Design review of the part built by this model. Coordinates are the model's own, in mm. A direction names the side the tool comes from. Round coordinates to 2 decimals unless told otherwise and drop trailing zeros. Write each loop counter-clockwise with the first axis right and the second up, starting at its lowest first coordinate (ties: lowest second). Pieces come first, ordered by that corner, then holes. Notation, with made-up numbers: M 35.25,30 L 86.25,30 A22 ccw 86.25,64 Z; hole C 32,4.5 d7. An arc over 180 degrees is marked long. One line per question, with ' | ' between items. Start each with the question number.
Item 1: Insertion check: pin 1 Ø2 at (y, z) = (23.5, -4) entering from +X; pin 2 Ø6 at (y, z) = (9.5, 12) entering from +X; pin 3 Ø3 at (y, z) = (3.5, 12.5) entering from -X. Each pin has a flat end and moves straight along its axis. Give the tip position at first contact, or say it passes through.
Item 2: For L1, parallel to Z at x = 7, y = 10; L2, parallel to Z at x = -12.5, y = 11; L3, parallel to X at y = 29, z = -7, list the stretches that pass through material, from the lowest coordinate up.
Item 3: Draft analysis for pull direction Z (two halves, no side actions). For faces 1 (the face through (27.5, 14, -16)), 2 (the face through (28, 19, 21)), 3 (the face through (7.454, 3, 4)), state which applies: released by +Z, released by -Z, zero draft, split by the parting line, or undercut.
Item 4: Add section A-A, the plane x = 0. State the section outline as (y, z) points, and give its area (3 significant figures).
Item 5: Machinability: for faces 4 (the face through (27.5, 14, 16)), 5 (the face through (7.454, 3, -26)), which of the approach directions +Z, -Z, +X, -X, +Y, -Y give a long, thin tool a straight path to every point of the face, cutting with its end or side? Answer none if there is none.
Item 6: Add section B-B, the plane z = 0. State the section outline as (x, y) points, and give its area (3 significant figures).
Item 7: Add section C-C, the plane x = -21. State the section outline as (y, z) points, and give its area (3 significant figures).
Item 8: Add section D-D, the plane y = 41. State the section outline as (x, z) points, and give its area (3 significant figures).
Autodesk Inventor part; units mm, degrees
ref_plane "YZ Plane" through (0, 0, 0) normal (1, 0, 0) x (0, 1, 0)
sketch "Sketch1" plane through (0, 0, 0) normal (0, 1, 0) x (-1, 0, 0)
  circle A0 centre (0, 0) radius 35
  dimension "d0" = 70
extrude "Extrusion1" add sketch "Sketch1" along normal blind 50
sketch "Sketch2" plane through (0, 0, 0) normal (1, 0, 0) x (0, 1, 0)
  point P0 (0, 0)
sketch "Sketch3" plane through (0, 0, 0) normal (0, 0, 1) x (1, 0, 0)
  line L0 (35, 50) -> (-35, 50)
  arc A0 (-35, 50) -> (35, 50) centre (0, 50) ccw
  point P0 (0, 0)
  dimension "d3" = 35
extrude "Extrusion2" cut sketch "Sketch3" against normal blind 50 and the other way blind 50
sketch "Sketch4" plane through (0, 0, 0) normal (0, 0, 1) x (1, 0, 0)
  arc A0 (7.4545, 6.2837) -> (-7.5, 5.4589) centre (0, 5.4589) ccw
  line L0 (7.4545, 6.2837) -> (7.4545, 0)
  line L1 (-35, 0) -> (35, 0)
  line L2 (-7.5, 5.4589) -> (-7.5, 0)
  line L3 (-7.5, 0) -> (7.4545, 0)
  line L4 (7.4545, 0) -> (3.6133, 0)
  line L5 (3.6133, 0) -> (-3.6133, 0)
  line L6 (-3.6133, 0) -> (-7.5, 0)
  point P0 (0, 0)
  dimension "d8" = 15
extrude "Extrusion3" cut sketch "Sketch4" along normal blind 50 and the other way blind 50
sketch "Sketch5" plane through (0, 0, 0) normal (0, 1, 0) x (-1, 0, 0)
  point P0 (0, 0)
sketch "Sketch6" plane through (0, 0, 0) normal (0, 1, 0) x (-1, 0, 0)
  line L0 (-27.5, -2) -> (27.5, -2)
  line L1 (27.5, -2) -> (27.5, 2)
  line L2 (27.5, 2) -> (-27.5, 2)
  line L3 (-27.5, 2) -> (-27.5, -2)
  line L4 (-27.5, -2) -> (27.5, 2) construction
  line L5 (27.5, -2) -> (-27.5, 2) construction
  line L6 (27.5, -6) -> (-27.5, -6)
  line L7 (-27.5, -6) -> (-27.5, -10)
  line L8 (-27.5, -10) -> (27.5, -10)
  line L9 (27.5, -10) -> (27.5, -6)
  line L10 (27.5, -14) -> (-27.5, -14)
  line L11 (-27.5, -14) -> (-27.5, -18)
  line L12 (-27.5, -18) -> (27.5, -18)
  line L13 (27.5, -18) -> (27.5, -14)
  line L14 (27.5, 10) -> (-27.5, 10)
  line L15 (-27.5, 10) -> (-27.5, 6)
  line L16 (-27.5, 6) -> (27.5, 6)
  line L17 (27.5, 6) -> (27.5, 10)
  line L18 (27.5, 2) -> (-27.5, 2)
  line L19 (-27.5, 2) -> (-27.5, -2)
  line L20 (-27.5, -2) -> (27.5, -2)
  line L21 (27.5, -2) -> (27.5, 2)
  line L22 (27.5, -6) -> (-27.5, -6)
  line L23 (-27.5, -6) -> (-27.5, -10)
  line L24 (-27.5, -10) -> (27.5, -10)
  line L25 (27.5, -10) -> (27.5, -6)
  line L26 (27.5, 18) -> (-27.5, 18)
  line L27 (-27.5, 18) -> (-27.5, 14)
  line L28 (-27.5, 14) -> (27.5, 14)
  line L29 (27.5, 14) -> (27.5, 18)
  line L30 (27.5, 10) -> (-27.5, 10)
  line L31 (-27.5, 10) -> (-27.5, 6)
  line L32 (-27.5, 6) -> (27.5, 6)
  line L33 (27.5, 6) -> (27.5, 10)
  line L34 (27.5, 2) -> (-27.5, 2)
  line L35 (-27.5, 2) -> (-27.5, -2)
  line L36 (-27.5, -2) -> (27.5, -2)
  line L37 (27.5, -2) -> (27.5, 2)
  point P0 (0, 0)
  dimension "d13" = 55
  dimension "d14" = 4
  dimension "d17" = 8
  dimension "d20" = 8
extrude "Extrusion4" cut sketch "Sketch6" along normal blind 50
properties part number "pipe_insert"
Computed values:
1) pin 1: stops at x = 34.87 | pin 2: stops at x = 33.82 | pin 3: stops at x = -33.23
2) L1: z = -34.29 to -18, -14 to -10, -6 to -2, 2 to 6, 10 to 14, 18 to 34.29 | L2: z = -32.69 to -18, -14 to -10, -6 to -2, 2 to 6, 10 to 14, 18 to 32.69 | L3: x = -34.29 to -28, 28 to 34.29
3) face 1: undercut | face 2: split by the parting line | face 3: zero draft
4) outline: M 12.96,-35 L 15,-35 L 15,-18 L 12.96,-18 Z; M 12.96,-14 L 15,-14 L 15,-10 L 12.96,-10 Z; M 12.96,-6 L 15,-6 L 15,-2 L 12.96,-2 Z; M 12.96,2 L 15,2 L 15,6 L 12.96,6 Z; M 12.96,10 L 15,10 L 15,14 L 12.96,14 Z; M 12.96,18 L 15,18 L 15,35 L 12.96,35 Z | area: 102 mm^2
5) face 4: +Y, -Y | face 5: +Z, -Z, -Y
6) outline: M -35,0 L -27.5,0 L -27.5,28.35 A35 cw -35,50 Z; M 27.5,0 L 35,0 L 35,50 A35 cw 27.5,28.35 Z | area: 528 mm^2
7) outline: M 0,-28 L 22,-28 L 22,-18 L 0,-18 Z; M 0,-14 L 22,-14 L 22,-10 L 0,-10 Z; M 0,-6 L 22,-6 L 22,-2 L 0,-2 Z; M 0,2 L 22,2 L 22,6 L 0,6 Z; M 0,10 L 22,10 L 22,14 L 0,14 Z; M 0,18 L 22,18 L 22,28 L 0,28 Z | area: 792 mm^2
8) outline: M -33.82,-9 L -33.82,9 A35 ccw Z; M 33.82,-9 A35 ccw 33.82,9 Z | area: 28.3 mm^2
